For this review, take the finished solid that the model builds, in its own axes (mm). Face numbers are marked on the shaded views. A direction names the side the tool comes from. Coordinates: 2 decimals unless noted, no trailing zeros. Order: outer loops, then holes, each group sorted by start corner. A loop starts at its lowest first (then second) coordinate and runs counter-clockwise, first axis right, second up. Notation, with made-up numbers: (56.25, 61.25) - (105.25, 61.25) arc R31 cw to (105.25, 93.25) - close; hole circle Ø3 at (-21.5, 56). An arc over 180 degrees is marked (long way). One line per item, written item: value. Start each with the question number.
(1) Mouldability with a two-part tool opening along Y and no side actions: class the marked faces 4, 5, 6 and 7 as released by +Y, released by -Y, zero draft, split by the parting line, or undercut.
(2) Consider section C-C on y = 7.5. Write out the cut boundary in (x, z), then the cut area to 3 significant figures.
(3) For the marked faces 1, 2 and 3, list the 3-axis set-ups (+Z, -Z, +X, -X, +Y, -Y) from which the entire face can be reached by the end or side of a thin tool; tool diameter is ignored.
(4) Consider section A-A on z = -4. Write out the cut boundary in (x, y), then the cut area to 3 significant figures.
(5) Clearance check with flat-ended pins moving along their axes: pin 1 (24 mm diameter, centred on x = 7.5, y = -2.5, fed in from +Z); pin 2 (5.5 mm diameter, centred on x = 36.5, z = -32.5, fed in from -Y); pin 3 (5.5 mm diameter, centred on y = -9.68, z = -54.39, fed in from +X); pin 4 (7.5 mm diameter, centred on x = 37, z = -23.5, fed in from +Y). State where each tip first meets the part, or that it passes through.
(6) To check wall thickness, follow line 1 along X through (y, z) = (10.5, -6.5); line 2 along Z through (x, y) = (12, 13); line 3 along Y through (x, z) = (-33.5, -15.5). State the ranges of each line that lie inside material, in increasing order.
(7) Consider section D-D on x = 18. Write out the cut boundary in (y, z), then the cut area to 3 significant figures.
(8) Consider section B-B on x = -2.5. Write out the cut boundary in (y, z).
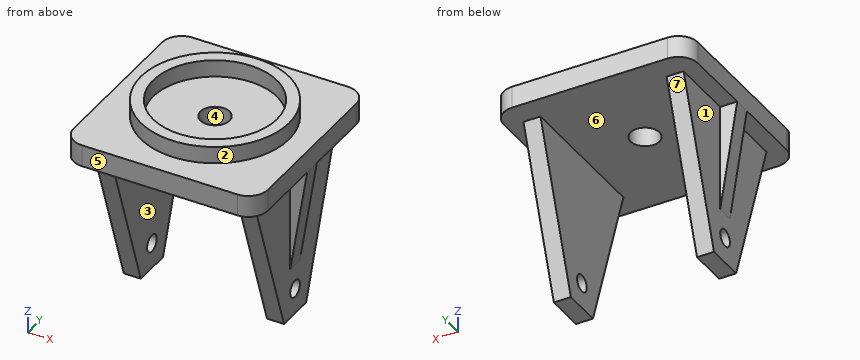
```python
from build123d import *

# Parameters (mm, degrees)
F1_DEPTH  = 9
F2_R      = 30.5
F2_R_2    = 25.5
F3_DEPTH  = 7
F4_R      = 6
F5_DEPTH  = 9.001
F6_W      = 7
F6_H      = 60
F7_DEPTH  = 65
F9_DEPTH  = 73.001
F11_DEPTH = 7
F13_DEPTH = 43.501
F15_DEPTH = 7
F17_DEPTH = 43.501
F18_R     = 3.5
F19_DEPTH = 73.001


with BuildPart() as f1:
    # F0 (on Top) → F1 (new body)
    with BuildSketch(Plane.XY):
        with BuildLine():
            Line((33.60959, 30.321302), (-30.39041, 30.321302))
            ThreePointArc((-30.39041, 30.321302), (-36.047264, 27.978156), (-38.39041, 22.321302))
            Line((-38.39041, 22.321302), (-38.39041, -41.678698))
            ThreePointArc((-38.39041, -41.678698), (-36.047264, -47.335552), (-30.39041, -49.678698))
            Line((-30.39041, -49.678698), (33.60959, -49.678698))
            ThreePointArc((33.60959, -49.678698), (39.266444, -47.335552), (41.60959, -41.678698))
            Line((41.60959, -41.678698), (41.60959, 22.321302))
            ThreePointArc((41.60959, 22.321302), (39.266444, 27.978156), (33.60959, 30.321302))
        make_face()
    extrude(amount=F1_DEPTH)

    # F2 (on face) → F3 (join)
    with BuildSketch(Plane.XY.offset(9)):
        with Locations((1.60959, -9.678698)):
            Circle(F2_R)
        with Locations((1.60959, -9.678698)):
            Circle(F2_R_2, mode=Mode.SUBTRACT)
    extrude(amount=F3_DEPTH)

    # F4 (on face) → F5 (cut, through all)
    with BuildSketch(Plane.XY.offset(9)):
        with Locations((1.60959, -9.678698)):
            Circle(F4_R)
    extrude(amount=-F5_DEPTH, mode=Mode.SUBTRACT)

    # F6 (on face) → F7 (join)
    with BuildSketch(Plane(origin=(0, 0, 0), x_dir=(1, 0, 0), z_dir=(0, 0, -1))):
        with Locations((-27.89041, 9.678698)):
            Rectangle(F6_W, F6_H)
        with Locations((31.10959, 9.678698)):
            Rectangle(F6_W, F6_H)
    extrude(amount=F7_DEPTH)

    # F8 (on face) → F9 (cut, through all)
    with BuildSketch(Plane.YZ.offset(34.60959)):
        Polygon((20.321302, -65), (20.321302, 0), (-1.678698, -65), align=None)
        Polygon((-17.678698, -65), (-39.678698, 0), (-39.678698, -65), align=None)
    extrude(amount=-F9_DEPTH, mode=Mode.SUBTRACT)

    # F10 (on face) → F11 (join)
    with BuildSketch(Plane.YZ.offset(34.60959)):
        Polygon((-6.178698, 0), (-9.678698, 0), (-13.178698, 0), (-13.178698, -44), (-6.178698, -44), align=None)
    extrude(amount=F11_DEPTH)

    # F12 (on face) → F13 (cut, through all)
    with BuildSketch(Plane(origin=(0, -6.178698, 0), x_dir=(-1, 0, 0), z_dir=(0, 1, 0))):
        Polygon((-34.60959, -44), (-41.60959, 0), (-41.60959, -44), align=None)
    extrude(amount=-F13_DEPTH, mode=Mode.SUBTRACT)

    # F14 (on face) → F15 (join)
    with BuildSketch(Plane(origin=(-31.39041, 0, 0), x_dir=(0, -1, 0), z_dir=(-1, 0, 0))):
        Polygon((13.178698, 0), (9.678698, 0), (6.178698, 0), (6.178698, -44), (13.178698, -44), align=None)
    extrude(amount=F15_DEPTH)

    # F16 (on face) → F17 (cut, through all)
    with BuildSketch(Plane.XZ.offset(13.178698)):
        Polygon((-31.39041, -44), (-38.39041, 0), (-38.39041, -44), align=None)
    extrude(amount=-F17_DEPTH, mode=Mode.SUBTRACT)

    # F18 (on face) → F19 (cut, through all)
    with BuildSketch(Plane.YZ.offset(34.60959)):
        with Locations((-9.678698, -54.387681)):
            Circle(F18_R)
    extrude(amount=-F19_DEPTH, mode=Mode.SUBTRACT)


solid = f1.part
```
Geometry check:
1. face 4: undercut
1. face 5: released by -Y
1. face 6: zero draft
1. face 7: released by +Y
2. outline: (-38.39, 0) - (-31.39, 0) - (-31.39, -37.88) - (-24.39, -37.88) - (-24.39, 0) - (27.61, 0) - (27.61, -37.88) - (34.61, -37.88) - (34.61, 0) - (41.61, 0) - (41.61, 9) - (26.81, 9) - (26.81, 16) - (20.45, 16) - (20.45, 9) - (-17.24, 9) - (-17.24, 16) - (-23.59, 16) - (-23.59, 9) - (-38.39, 9) - close
2. area: 1,340 mm^2
3. face 1: -Z, -X
3. face 2: +Z
3. face 3: -Z, +Y, -Y
4. outline: (-37.75, -13.18) - (-31.39, -13.18) - (-31.39, -38.32) - (-24.39, -38.32) - (-24.39, 18.97) - (-31.39, 18.97) - (-31.39, -6.18) - (-37.75, -6.18) - close; (27.61, -38.32) - (34.61, -38.32) - (34.61, -13.18) - (40.97, -13.18) - (40.97, -6.18) - (34.61, -6.18) - (34.61, 18.97) - (27.61, 18.97) - close
4. area: 891 mm^2
5. pin 1: stops at z = 9
5. pin 2: stops at y = -29.35
5. pin 3: passes through
5. pin 4: stops at y = 13.35
6. line 1: x = -31.39 to -24.39, 27.61 to 34.61
6. line 2: z = 0 to 9
6. line 3: y = -13.18 to -6.18
7. outline: (-49.68, 0) - (30.32, 0) - (30.32, 9) - (16.04, 9) - (16.04, 16) - (9.86, 16) - (9.86, 9) - (-29.21, 9) - (-29.21, 16) - (-35.4, 16) - (-35.4, 9) - (-49.68, 9) - close
7. area: 807 mm^2
8. outline: (-49.68, 0) - (-14.05, 0) - (-14.05, 9) - (-34.85, 9) - (-34.85, 16) - (-39.9, 16) - (-39.9, 9) - (-49.68, 9) - close; (-5.31, 0) - (30.32, 0) - (30.32, 9) - (20.54, 9) - (20.54, 16) - (15.49, 16) - (15.49, 9) - (-5.31, 9) - close
